```python
from build123d import *

# Parameters (mm, degrees)
SKETCH1_W           = 42
SKETCH1_H           = 42
BOSS_EXTRUDE1_DEPTH = 40
SKETCH2_R           = 11
SKETCH2_R_2         = 5
BOSS_EXTRUDE2_DEPTH = 2
BOSS_EXTRUDE3_DEPTH = 23
SKETCH4_R           = 1.5
CUT_EXTRUDE1_DEPTH  = 2.68
SKETCH5_R           = 3
CUT_EXTRUDE2_DEPTH  = 2.68
SKETCH6_R           = 5
CUT_EXTRUDE3_DEPTH  = 2.68
SKETCH7_R           = 3.5
SKETCH7_R_2         = 3.4238
SKETCH7_R_3         = 2.5
SKETCH7_R_4         = 2.4238
CUT_EXTRUDE4_DEPTH  = 0.0254
CHAMFER1_SIZE       = 3.81
SKETCH8_W           = 2.5
SKETCH8_H           = 16
BOSS_EXTRUDE4_DEPTH = 4
SKETCH9_W           = 6
SKETCH9_H           = 16
SKETCH9_W_2         = 5.8476
SKETCH9_H_2         = 15.8476
CUT_EXTRUDE5_DEPTH  = 0.0254
SKETCH10_W          = 0.508
SKETCH10_H          = 0.508
BOSS_EXTRUDE5_DEPTH = 6


with BuildPart() as part:
    # Sketch1 → Boss-Extrude1 (new body)
    with BuildSketch(Plane.XY):
        with Locations((21, -21)):
            Rectangle(SKETCH1_W, SKETCH1_H)
    extrude(amount=BOSS_EXTRUDE1_DEPTH)

    # Sketch2 → Boss-Extrude2 (add)
    with BuildSketch(Plane.XY.offset(40)):
        with Locations((21, -21)):
            Circle(SKETCH2_R)
        with Locations((21, -21)):
            Circle(SKETCH2_R_2, mode=Mode.SUBTRACT)
    extrude(amount=BOSS_EXTRUDE2_DEPTH)

    # Sketch3 → Boss-Extrude3 (add)
    with BuildSketch(Plane.XY.offset(40)):
        with BuildLine():
            Line((23.063065241, -21.897920826), (22.998678024, -19.966662613))
            ThreePointArc((22.998678024, -19.966662613), (18.751249422, -21.074972259), (23.063065241, -21.897920826))
        make_face()
    extrude(amount=BOSS_EXTRUDE3_DEPTH)

    # Sketch4 → Cut-Extrude1 (cut)
    with BuildSketch(Plane.XY.offset(40)):
        with Locations((5, -5)):
            Circle(SKETCH4_R)
        with Locations((5, -37)):
            Circle(SKETCH4_R)
        with Locations(Location((37, -5, 0), (0, 0, 180))):
            Circle(SKETCH4_R)
        with Locations(Location((37, -37, 0), (0, 0, 180))):
            Circle(SKETCH4_R)
    extrude(amount=-CUT_EXTRUDE1_DEPTH, mode=Mode.SUBTRACT)

    # Sketch5 → Cut-Extrude2 (cut)
    with BuildSketch(Plane(origin=(0, 0, 0), x_dir=(-1, 0, 0), z_dir=(0, 0, -1))):
        with Locations((-37, -5)):
            Circle(SKETCH5_R)
        with Locations((-37, -37)):
            Circle(SKETCH5_R)
        with Locations(Location((-5, -37, 0), (0, 0, 180))):
            Circle(SKETCH5_R)
        with Locations(Location((-5, -5, 0), (0, 0, 180))):
            Circle(SKETCH5_R)
    extrude(amount=-CUT_EXTRUDE2_DEPTH, mode=Mode.SUBTRACT)

    # Sketch6 → Cut-Extrude3 (cut)
    with BuildSketch(Plane(origin=(0, 0, 0), x_dir=(-1, 0, 0), z_dir=(0, 0, -1))):
        with Locations(Location((-21, -21, 0), (0, 0, 180))):
            Circle(SKETCH6_R)
    extrude(amount=-CUT_EXTRUDE3_DEPTH, mode=Mode.SUBTRACT)

    # Sketch7 → Cut-Extrude4 (cut)
    # profile 1 of 2: a face of its own
    with BuildSketch(Plane(origin=(0, 0, 2.68), x_dir=(-1, 0, 0), z_dir=(0, 0, -1))):
        with Locations((-21, -21)):
            Circle(SKETCH7_R)
        with Locations((-21, -21)):
            Circle(SKETCH7_R_2, mode=Mode.SUBTRACT)
    # profile 2 of 2: a face of its own
    with BuildSketch(Plane(origin=(0, 0, 2.68), x_dir=(-1, 0, 0), z_dir=(0, 0, -1))):
        with Locations((-21, -21)):
            Circle(SKETCH7_R_3)
        with Locations((-21, -21)):
            Circle(SKETCH7_R_4, mode=Mode.SUBTRACT)
    extrude(amount=-CUT_EXTRUDE4_DEPTH, mode=Mode.SUBTRACT)

    # Chamfer1
    chamfer1_edges = [part.edges().sort_by_distance(p)[0] for p in [
        (0, 0, 20),
        (42, 0, 20),
        (42, -42, 20),
        (0, -42, 20),
    ]]
    chamfer(chamfer1_edges, length=CHAMFER1_SIZE)

    # Sketch8 → Boss-Extrude4 (add)
    with BuildSketch(Plane(origin=(42, 0, 0), x_dir=(0, 0, -1), z_dir=(1, 0, 0))):
        with Locations((-1.25, -20.954)):
            Rectangle(SKETCH8_W, SKETCH8_H)
    extrude(amount=BOSS_EXTRUDE4_DEPTH)

    # Sketch9 → Cut-Extrude5 (cut)
    with BuildSketch(Plane(origin=(42, 0, 0), x_dir=(0, 0, -1), z_dir=(1, 0, 0))):
        with Locations((-5.5, -20.954)):
            Rectangle(SKETCH9_W, SKETCH9_H)
        with Locations((-5.5, -20.954)):
            Rectangle(SKETCH9_W_2, SKETCH9_H_2, mode=Mode.SUBTRACT)
    extrude(amount=-CUT_EXTRUDE5_DEPTH, mode=Mode.SUBTRACT)

    # Sketch10 → Boss-Extrude5 (add)
    with BuildSketch(Plane(origin=(42, 0, 0), x_dir=(0, 0, -1), z_dir=(1, 0, 0))):
        Polygon((-7.9158, -28.3698), (-7.9158, -26.311363573), (-8.4238, -26.311363573), (-8.4238, -28.8778), (-2.5762, -28.8778), (-2.5762, -13.0302), (-8.4238, -13.0302), (-8.4238, -15.827398032), (-7.9158, -15.827398032), (-7.9158, -13.5382), (-3.0842, -13.5382), (-3.0842, -28.3698), align=None)
        with Locations((-6.058218613, -24.450923399)):
            Rectangle(SKETCH10_W, SKETCH10_H)
        with Locations((-6.058218613, -26.990923399)):
            Rectangle(SKETCH10_W, SKETCH10_H)
        with Locations((-6.058218613, -21.910923399)):
            Rectangle(SKETCH10_W, SKETCH10_H)
        with Locations((-6.058218613, -19.370923399)):
            Rectangle(SKETCH10_W, SKETCH10_H)
        with Locations((-6.058218613, -16.830923399)):
            Rectangle(SKETCH10_W, SKETCH10_H)
        with Locations((-6.058218613, -14.290923399)):
            Rectangle(SKETCH10_W, SKETCH10_H)
    extrude(amount=BOSS_EXTRUDE5_DEPTH)


solid = part.part
```
The listing builds one solid part. Answer for the finished solid, in the listing's coordinates (mm). A direction names the side the tool comes from. Coordinates: 2 decimals unless noted, no trailing zeros. Loops run counter-clockwise (first coordinate to the right, second up) from the corner with the lowest first, then second, coordinate; pieces in that order, holes last. Notation, with made-up numbers: M 14.25,75.25 L 72.25,75.25 A18 cw 72.25,82.25 Z; hole C -24,75 d2. An arc over 180 degrees is marked long. Answer as CSV lines item,"result". Start each with the question number.
(1) For faces 5 (the flat face through (45, -13.03, 5)), 6 (the flat face through (45, -27, 7.916)), 7 (the cylindrical face through (4.675, -38.464, 38.679)), 8 (the cylindrical face through (4.35, -2.07, 1.32)), determine the directions among +Z, -Z, +X, -X, +Y, -Y from which every point of the face is accessible in a straight line to the end or side of a thin tool.
(2) Find the intervals of material crossed by L1, parallel to Y at x = 5, z = 39; L2, parallel to Y at x = 5, z = 1.05; L3, parallel to Y at x = 46.5, z = 7.5, in increasing order. Write a range as [from, to].
(3) The part is cut by section C-C (x = 37). Give the vertices of the cut face in (y, z), and give its area (3 significant figures).
(4) The mould has two halves that part along X. Classify faces 1 (the flat face through (45, -15, 7.916)), 2 (the cylindrical face through (38.2, -4.1, 38.7)), 3 (the flat face through (37, -37, 2.68)), 4 (the flat face through (0, -21, 20)): pulls with the +X half, pulls with the -X half, needs draft (parallel to the pull), parting line crosses it, or undercut.
(5) The part is cut by section B-B (z = 13.5). Give the vertices of the cut face in (x, y), and give its area (3 significant figures).
(6) Given pin 1 (2.5 mm diameter, centred on x = 5, y = -5, fed in from +Z); pin 2 (1.5 mm diameter, centred on x = 14.5, y = -18.5, fed in from +Z); pin 3 (5 mm diameter, centred on x = 7, y = -16.5, fed in from +Z); pin 4 (1.8 mm diameter, centred on x = 45, y = -15, fed in from -Z), each flat-ended and moving along its own axis, determine where each tip first touches the part or whether it passes through.
(7) The part is cut by section A-A (y = -5). Give the vertices of the cut face in (x, z), and give its area (3 significant figures).
(8) The part is cut by section D-D (y = -30). Give the vertices of the cut face in (x, z).
Determined:
1,face 5,"+Z, +X, +Y"
1,face 6,"+X"
1,face 7,"+Z"
1,face 8,"-Z"
2,L1,"[-42, -38.5], [-35.5, -6.5], [-3.5, 0]"
2,L2,"[-42, -40], [-34, -8], [-2, 0]"
2,L3,"[-28.88, -28.37], [-13.54, -13.03]"
3,outline,"M -42,0 L -40,0 L -40,2.68 L -34,2.68 L -34,0 L -8,0 L -8,2.68 L -2,2.68 L -2,0 L 0,0 L 0,40 L -3.5,40 L -3.5,37.32 L -6.5,37.32 L -6.5,40 L -35.5,40 L -35.5,37.32 L -38.5,37.32 L -38.5,40 L -42,40 Z"
3,area,"1,630 mm2"
4,face 1,"needs draft"
4,face 2,"undercut"
4,face 3,"undercut"
4,face 4,"pulls with the -X half"
5,outline,"M 0,-38.19 L 3.81,-42 L 38.19,-42 L 42,-38.19 L 42,-3.81 L 38.19,0 L 3.81,0 L 0,-3.81 Z"
5,area,"1,730 mm2"
6,pin 1,"z = 37.32"
6,pin 2,"z = 42"
6,pin 3,"z = 40"
6,pin 4,"z = 0"
7,outline,"M 0,0 L 2,0 L 2,2.68 L 8,2.68 L 8,0 L 34,0 L 34,2.68 L 40,2.68 L 40,0 L 42,0 L 42,40 L 38.5,40 L 38.5,37.32 L 35.5,37.32 L 35.5,40 L 6.5,40 L 6.5,37.32 L 3.5,37.32 L 3.5,40 L 0,40 Z"
7,area,"1,630 mm2"
8,outline,"M 0,0 L 42,0 L 42,40 L 27.32,40 L 27.32,42 L 14.68,42 L 14.68,40 L 0,40 Z"
